Job drawing, mm, ordinate dimensions from the low corner. One solid piece. A direction names the side the tool comes from. Give positions to 0.01 mm unless a question says otherwise; leave off trailing zeros. Order: outer loops, then holes, each group sorted by start corner. A loop starts at its lowest first (then second) coordinate and runs counter-clockwise, first axis right, second up. Notation, with made-up numbers: (-35.75, 3.5) -> (-25.75, 3.5) arc R29 cw to (-25.75, 26.5) -> close; hole circle Ø8 at (44.5, 43.5). An arc over 180 degrees is marked (long way). Use CSV: the item, a comma, the result in double quotes. Start each with the question number.
1. Drop flat-ended pins along their axis: pin 1 (1.6 mm diameter, centred on x = 3, z = 2, fed in from -Y); pin 2 (1 mm diameter, centred on y = 18.5, z = 5, fed in from +X); pin 3 (3.5 mm diameter, centred on x = 4.5, z = 2.5, fed in from +Y). Give the stop position or say it passes through.
2. Cut at A-A on y = 14.75. List the corners of the cut face in (x, z), then the cut area to 3 significant figures.
3. Wall check: line 1 (Y direction, x = 7, z = 5.25); line 2 (Y direction, x = 2, z = 2.25); line 3 (X direction, y = 10.75, z = 0.5). Give the ranges that are in metal, low to high. Write a range as from..to.
4. Pull direction X, two halves, no side cores. Call the marked faces 4, 5 and 6: released by +X, released by -X, zero draft, split by the parting line, or undercut.
5. 3-axis set-ups, long thin cutter, end or side, ignore diameter. For the marked faces 1, 2 and 3: which of +Z, -Z, +X, -X, +Y, -Y reach the whole face in a straight line?
6. Cut at B-B on x = 1.75. List the corners of the cut face in (y, z).
7. Cut at C-C on z = 0.75. List the corners of the cut face in (x, y), then the cut area to 3 significant figures.
8. Cut at D-D on y = 17.75. List the corners of the cut face in (x, z), then the cut area to 3 significant figures.
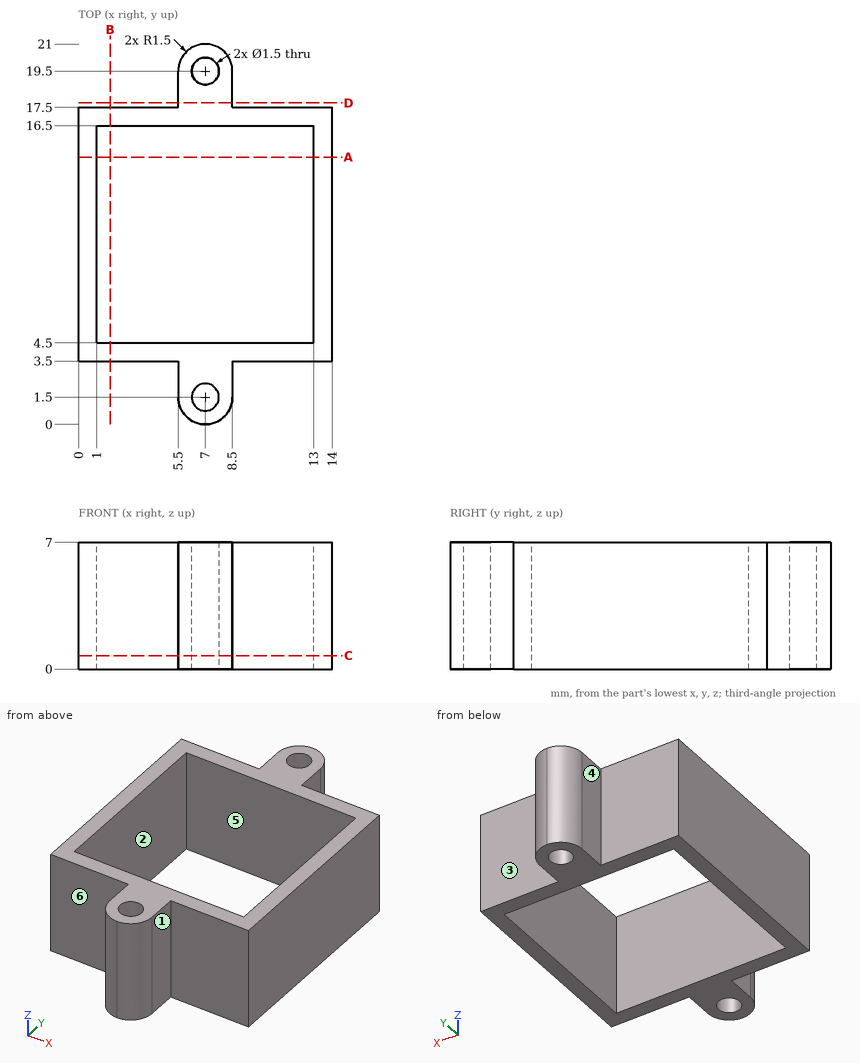
Verdict:
1,pin 1,"y = 3.5"
1,pin 2,"x = 8.5"
1,pin 3,"y = 20.8"
2,outline,"(0, 0) -> (1, 0) -> (1, 7) -> (0, 7) -> close; (13, 0) -> (14, 0) -> (14, 7) -> (13, 7) -> close"
2,area,"14.0 mm^2"
3,line 1,"0..0.75, 2.25..4.5, 16.5..18.75, 20.25..21"
3,line 2,"3.5..4.5, 16.5..17.5"
3,line 3,"0..1, 13..14"
4,face 4,"released by -X"
4,face 5,"undercut"
4,face 6,"zero draft"
5,face 1,"+Z, -Z, +X, -Y"
5,face 2,"+Z, -Z"
5,face 3,"+Z, -Z, +X, +Y"
6,outline,"(3.5, 0) -> (4.5, 0) -> (4.5, 7) -> (3.5, 7) -> close; (16.5, 0) -> (17.5, 0) -> (17.5, 7) -> (16.5, 7) -> close"
7,outline,"(0, 3.5) -> (5.5, 3.5) -> (5.5, 1.5) arc R1.5 ccw to (8.5, 1.5) -> (8.5, 3.5) -> (14, 3.5) -> (14, 17.5) -> (8.5, 17.5) -> (8.5, 19.5) arc R1.5 ccw to (5.5, 19.5) -> (5.5, 17.5) -> (0, 17.5) -> close; hole (1, 4.5) -> (13, 4.5) -> (13, 16.5) -> (1, 16.5) -> close; hole circle Ø1.5 at (7, 1.5); hole circle Ø1.5 at (7, 19.5)"
7,area,"67.5 mm^2"
8,outline,"(5.5, 0) -> (8.5, 0) -> (8.5, 7) -> (5.5, 7) -> close"
8,area,"21.0 mm^2"
